Here's the drawing with two shaded views (mm, measured from the low corner). I have some questions. Give positions to 0.01 mm unless a question says otherwise; leave off trailing zeros. Loops run counter-clockwise (first coordinate to the right, second up) from the corner with the lowest first, then second, coordinate; pieces in that order, holes last.
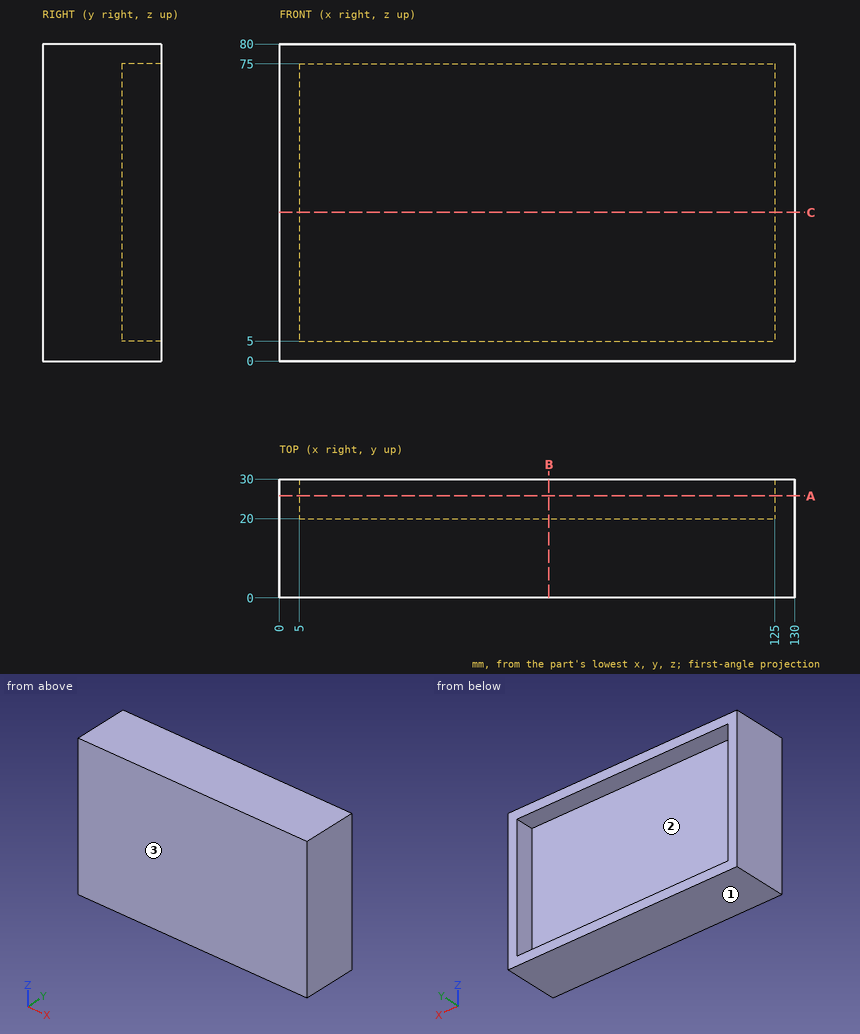
(1) Will this pin go through, and if not, where does the flat tip stop? P1, Ø3, axis at y = 8, z = 38, coming from the -X side.
Returned:
P1: stops at x = 0
(2) Suppose I cut it at C-C on z = 37.5. List the corners of the cut face in (x, y) for me.
Returned:
outline: (0, 0) - (130, 0) - (130, 30) - (125, 30) - (125, 20) - (5, 20) - (5, 30) - (0, 30) - close
(3) Thinking about a two-plate mould opening in Z: for the marked faces 1, 2 and 3, which applies, pulls with the +Z half, pulls with the -Z half, needs draft (parallel to the pull), parting line crosses it, or undercut?
Returned:
face 1: pulls with the -Z half
face 2: undercut
face 3: needs draft
(4) Suppose I cut it at B-B on x = 68. List the corners of the cut face in (y, z) for me.
Returned:
outline: (0, 0) - (30, 0) - (30, 5) - (20, 5) - (20, 75) - (30, 75) - (30, 80) - (0, 80) - close
(5) Please list where these lines run through material, in increasing order: probe 1 along X at (y, z) = (25, 11); probe 2 along Z at (x, y) = (85, 25.25); probe 3 along Y at (x, z) = (95, 71).
Returned:
probe 1: x = 0 to 5, 125 to 130
probe 2: z = 0 to 5, 75 to 80
probe 3: y = 0 to 20
(6) Suppose I cut it at A-A on y = 25.75. List the corners of the cut face in (x, z) for me.
Returned:
outline: (0, 0) - (130, 0) - (130, 80) - (0, 80) - close; hole (5, 5) - (125, 5) - (125, 75) - (5, 75) - close
